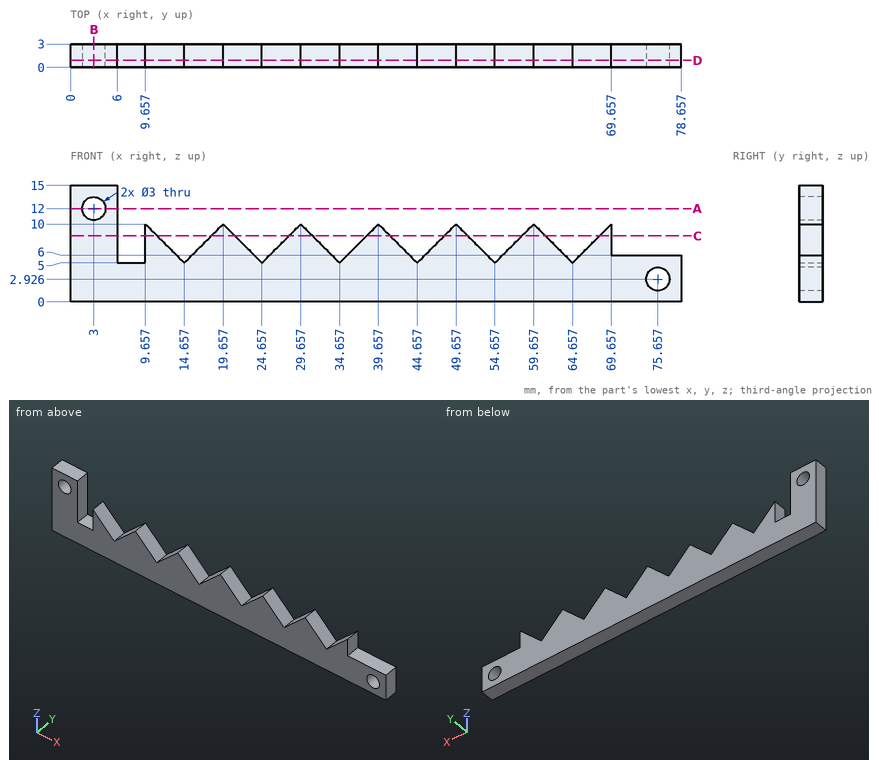
The drawing under review shows one solid part. Ordinate dimensions are in mm from its lowest x, y, z. Coordinates: 2 decimals unless noted, no trailing zeros. Write each loop counter-clockwise with the first axis right and the second up, starting at its lowest first coordinate (ties: lowest second). Pieces come first, ordered by that corner, then holes. Notation, with made-up numbers: M 17.5,-39.5 L 64.5,-39.5 A31 cw 64.5,-1.5 Z; hole C 40.5,68.25 d11. An arc over 180 degrees is marked long. Answer as a JSON object with one key per item and string values.
Item 1: Insertion check: pin 1 Ø0.9 at (y, z) = (1, 8.5) entering from +X; pin 2 Ø5 at (x, z) = (41, 7.5) entering from -Y; pin 3 Ø2.5 at (x, z) = (75.66, 2.93) entering from -Y. Each pin has a flat end and moves straight along its axis. Give the tip position at first contact, or say it passes through.
Outcome:
{"pin 1": "x = 69.66", "pin 2": "y = 0", "pin 3": "through"}
Item 2: Add section C-C, the plane z = 8.5. State how many separate pieces and enclosed holes the cut face has, and give its area (3 significant figures).
Outcome:
{"separate pieces": "8", "enclosed holes": "0", "area": "72.0 mm²"}
Item 3: Add section B-B, the plane x = 3. Give the boundary of the cut face in (y, z).
Outcome:
{"outline": "M 0,0 L 3,0 L 3,10.5 L 0,10.5 Z; M 0,13.5 L 3,13.5 L 3,15 L 0,15 Z"}
Item 4: Add section A-A, the plane z = 12. Give the boundary of the cut face in (x, y).
Outcome:
{"outline": "M 0,0 L 1.5,0 L 1.5,3 L 0,3 Z; M 4.5,0 L 6,0 L 6,3 L 4.5,3 Z"}
Item 5: Wall thickness on probe 1 along X at (y, z) = (0.9, 12); probe 2 along Z at (x, y) = (3, 1.7); probe 3 along X at (y, z) = (1.65, 3) (1 decimal): over which ranges is each line inside the solid? List them lowest first.
Outcome:
{"probe 1": "0 to 1.5, 4.5 to 6", "probe 2": "0 to 10.5, 13.5 to 15", "probe 3": "0 to 74.2, 77.2 to 78.7"}
Item 6: Add section D-D, the plane y = 0.9. Give the boundary of the cut face in (x, z).
Outcome:
{"outline": "M 0,0 L 78.66,0 L 78.66,6 L 69.66,6 L 69.66,10 L 64.66,5 L 59.66,10 L 54.66,5 L 49.66,10 L 44.66,5 L 39.66,10 L 34.66,5 L 29.66,10 L 24.66,5 L 19.66,10 L 14.66,5 L 9.66,10 L 9.66,5 L 6,5 L 6,15 L 0,15 Z; hole C 3,12 d3; hole C 75.66,2.93 d3"}
